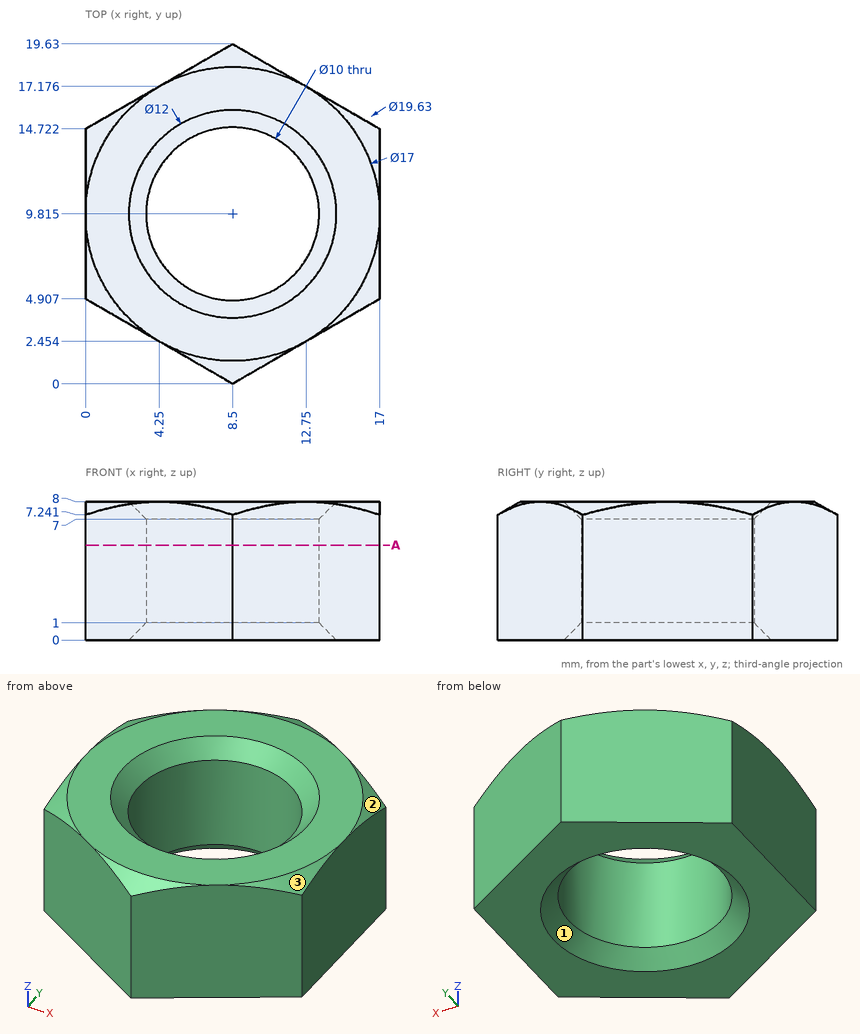
Geometry: see drawing. Coordinates: mm, zero at the bounding-box minimum. Give positions to 0.01 mm unless a question says otherwise; leave off trailing zeros. Write each loop counter-clockwise with the first axis right and the second up, starting at its lowest first coordinate (ties: lowest second). Pieces come first, ordered by that corner, then holes. Notation, with made-up numbers: M 43,31 L 52,31 A18 ccw 52,59 Z; hole C 8.25,3.25 d1. An arc over 180 degrees is marked long. Answer in a Markdown table with one row per item. Add a question column.
(1) First-contact query: pin 1 (9 mm diameter, centred on x = 8.5, y = 9.81, fed in from -Z). Flat tip, straight axial feed; report the tip coordinate or a pass-through.
(2) Ray query, line 1 (X direction, y = 11, z = 1.5); line 2 (Y direction, x = 9.75, z = 1.25) (1 decimal); line 3 (X direction, y = 12, z = 1.75). Return the intervals inside material, ascending.
(3) Section A-A on z = 5.5. Return loops of the section in (x, y) (1 decimal), and give its area (3 significant figures).
(4) Mould query, pull axis Y, two halves, no side actions, for the marked faces 1, 2 and 3. Classes: +Y half, -Y half, draft (parallel to the pull), parting line (faces both ways), or undercut.
Result set:
| question | item | result |
|---|---|---|
| 1 | pin 1 | passes through |
| 2 | line 1 | x = 0 to 3.64, 13.36 to 17 |
| 2 | line 2 | y = 0.7 to 5, 14.7 to 18.9 |
| 2 | line 3 | x = 0 to 4, 13 to 17 |
| 3 | outline | M 0,4.9 L 8.5,0 L 17,4.9 L 17,14.7 L 8.5,19.6 L 0,14.7 Z; hole C 8.5,9.8 d10 |
| 3 | area | 172 mm^2 |
| 4 | face 1 | undercut |
| 4 | face 2 | +Y half |
| 4 | face 3 | -Y half |
